```python
from build123d import *

# Parameters (mm, degrees)
F1_DEPTH = 15
F3_W     = 43.98863
F3_H     = 20
F4_DEPTH = 1.2
F2_R     = 4.75
F5_DEPTH = 1.21
F6_R     = 1.385
F7_DEPTH = 1.2


with BuildPart() as f1:
    # F0 (on Right) → F1 (new body, symmetric)
    with BuildSketch(Plane.YZ):
        Polygon((-116.29, 12.5), (-117.5, 12.5), (-117.5, -12.5), (117.5, -12.5), (117.5, 12.5), (116.29, 12.5), (116.29, -11.29), (0, -11.29), (-116.29, -11.29), align=None)
    extrude(amount=F1_DEPTH, both=True)

    # F3 (on face) → F4 (join)
    with BuildSketch(Plane.YZ.offset(15)):
        with Locations((-94.194315, -2.5)):
            Rectangle(F3_W, F3_H)
        with Locations((94.194315, -2.5)):
            Rectangle(F3_W, F3_H)
    extrude(amount=F4_DEPTH)

    # F2 (on face) → F5 (cut, through all)
    with BuildSketch(Plane(origin=(0, 117.5, 0), x_dir=(-1, 0, 0), z_dir=(0, 1, 0))):
        Circle(F2_R)
    extrude(amount=-F5_DEPTH, mode=Mode.SUBTRACT)

    # F6 (on face) → F7 (cut, through all)
    with BuildSketch(Plane.YZ.offset(16.2)):
        with Locations((-77.616818, -5)):
            Circle(F6_R)
        with Locations((77.616818, -5)):
            Circle(F6_R)
    extrude(amount=-F7_DEPTH, mode=Mode.SUBTRACT)


solid = f1.part
```
Part model, mm, in its own coordinate system. A direction names the side the tool comes from. Give positions to 0.01 mm unless a question says otherwise; leave off trailing zeros. Loops run counter-clockwise (first coordinate to the right, second up) from the corner with the lowest first, then second, coordinate; pieces in that order, holes last. Notation, with made-up numbers: M 16,57 L 70,57 A9 cw 70,70 Z; hole C -26,-21.75 d7. An arc over 180 degrees is marked long. Return JSON: item names as keys, results as strings.
1) Drill centre lines: line 1 (Y direction, x = -9.5, z = -3.5); line 2 (Z direction, x = -5.5, y = 105); line 3 (X direction, y = 106, z = 2.5). Where is each one in solid material? Low to high.
Calculated:
{"line 1": "y = -117.5 to -116.29, 116.29 to 117.5", "line 2": "z = -12.5 to -11.29", "line 3": "x = 15 to 16.2"}
2) Flat gauge pins, fed straight in: pin 1 Ø1 at (y, z) = (-13, -12) entering from +X; pin 2 Ø15 at (y, z) = (92, 1) entering from -X; pin 3 Ø2 at (y, z) = (54, -9) entering from -X; pin 4 Ø1 at (x, y) = (15.5, 98) entering from +Z. Where does each tip first touch, or does it go through?
Calculated:
{"pin 1": "stops at x = 15", "pin 2": "stops at x = 15", "pin 3": "passes through", "pin 4": "stops at z = 7.5"}
3) Saw through at D-D, the plane x = -12. List the corners of the cut face in (y, z), then the cut area to 3 significant figures.
Calculated:
{"outline": "M -117.5,-12.5 L 117.5,-12.5 L 117.5,12.5 L 116.29,12.5 L 116.29,-11.29 L -116.29,-11.29 L -116.29,12.5 L -117.5,12.5 Z", "area": "342 mm2"}
4) Pull direction Z, two halves, no side cores. Call faces 1 (the face through (0, -2, -12.5)), 2 (the face through (16.2, -95, -2)), 3 (the face through (0, 2, -11.29)), 4 (the face through (-2.192, 116.903, -4.214)): released by +Z, released by -Z, zero draft, split by the parting line, or undercut.
Calculated:
{"face 1": "released by -Z", "face 2": "zero draft", "face 3": "released by +Z", "face 4": "undercut"}
5) Saw through at A-A, the plane x = 0. List the corners of the cut face in (y, z).
Calculated:
{"outline": "M -117.5,-12.5 L 117.5,-12.5 L 117.5,-4.75 L 116.29,-4.75 L 116.29,-11.29 L -116.29,-11.29 L -116.29,12.5 L -117.5,12.5 Z; M 116.29,4.75 L 117.5,4.75 L 117.5,12.5 L 116.29,12.5 Z"}
6) Saw through at C-C, the plane y = -101. List the corners of the cut face in (x, z).
Calculated:
{"outline": "M -15,-12.5 L 16.2,-12.5 L 16.2,7.5 L 15,7.5 L 15,-11.29 L -15,-11.29 Z"}
7) 3-axis set-ups, long thin cutter, end or side, ignore diameter. For faces 5 (the face through (16.2, 94, -2)), 6 (the face through (15, -95, -2)): which of +Z, -Z, +X, -X, +Y, -Y reach the whole face in a straight line?
Calculated:
{"face 5": "+Z, -Z, +X, +Y, -Y", "face 6": "+Z, -X"}
8) Saw through at B-B, the plane z = 0. List the corners of the cut face in (x, y).
Calculated:
{"outline": "M -15,-117.5 L 15,-117.5 L 15,-116.29 L -15,-116.29 Z; M -15,116.29 L -4.75,116.29 L -4.75,117.5 L -15,117.5 Z; M 4.75,116.29 L 15,116.29 L 15,117.5 L 4.75,117.5 Z; M 15,-116.19 L 16.2,-116.19 L 16.2,-72.2 L 15,-72.2 Z; M 15,72.2 L 16.2,72.2 L 16.2,116.19 L 15,116.19 Z"}
